CAD build for the part. Positions are in the model's coordinates, mm. Face numbers are marked on the shaded views. A direction names the side the tool comes from. Give positions to 0.01 mm unless a question says otherwise; leave off trailing zeros. Write each loop counter-clockwise with the first axis right and the second up, starting at its lowest first coordinate (ties: lowest second). Pieces come first, ordered by that corner, then holes. Notation, with made-up numbers: (6.25, 81) - (56.25, 81) arc R11 cw to (56.25, 93) - close; hole circle Ø6 at (-38, 76.25). An arc over 180 degrees is marked (long way). Put each result on its own line as item: value. Start each with the question number.
1. Mould opens along X. For the marked faces 4 and 5 say: +X half, -X half, draft (parallel to the pull), parting line (faces both ways), or undercut.
2. Tool access for the marked faces 1, 2 and 3: list every direction of +Z, -Z, +X, -X, +Y, -Y with a clear straight run to the whole face (end or side of a thin tool).
3. Cut at B-B on y = -24.45. List the corners of the cut face in (x, z).
4. Cut at C-C on x = 1.5. List the corners of the cut face in (y, z).
5. Cut at D-D on z = 9.5. List the corners of the cut face in (x, y), and give its area (3 significant figures).
6. Wall check: line 1 (X direction, y = -11.9, z = 1.75); line 2 (X direction, y = -46, z = 8.5); line 3 (X direction, y = -33.25, z = 1.55). Give the ranges that are in metal, low to high.
7. Cut at A-A on z = 16.5. List the corners of the cut face in (x, y).
8. Drop flat-ended pins along their axis: pin 1 (9.5 mm diameter, centred on x = 0, y = -52.1, fed in from -Z); pin 2 (1 mm diameter, centred on x = 17, z = 11.5, fed in from +Y); pin 3 (0.8 mm diameter, centred on y = -49.5, z = 2, fed in from +X); pin 4 (3 mm diameter, centred on x = -23.5, y = -24.45, fed in from -Z). Give the stop position or say it passes through.
Autodesk Inventor part; units mm, degrees
ref_plane "YZ Plane" through (0, 0, 0) normal (1, 0, 0) x (0, 1, 0)
ref_plane "XZ Plane" through (0, 0, 0) normal (0, 1, 0) x (-1, 0, 0)
ref_plane "XY Plane" through (0, 0, 0) normal (0, 0, 1) x (1, 0, 0)
sketch "Sketch1" plane through (0, 0, 0) normal (0, 0, 1) x (1, 0, 0)
  line L0 (-20, 0) -> (20, 0)
  line L1 (32, -12) -> (32, -47.5)
  line L2 (0, -64) -> (0, -64)
  line L3 (-32, -47.5) -> (-32, -12)
  arc A0 (-20, 0) -> (-32, -12) centre (-20, -12) ccw
  arc A1 (32, -12) -> (20, 0) centre (20, -12) ccw
  line L4 (-12, -52) -> (-12, -47.5)
  line L5 (-12, -47.5) -> (-32, -47.5)
  line L6 (12, -52) -> (12, -47.5)
  line L7 (12, -47.5) -> (32, -47.5)
  circle A2 centre (0, -52.1) radius 3.6
  line L8 (0, -80.2794) -> (0, 16.2794)
  arc A3 (-12, -52) -> (0, -64) centre (0, -52) ccw
  arc A4 (0, -64) -> (12, -52) centre (0, -52) ccw
  point P0 (0, 0)
  point P1 (0, 0)
  point P2 (0, -64)
  dimension "d0" = 64
  dimension "d1" = 64
  dimension "d2" = 12
  dimension "d3" = 47.5
  dimension "d4" = 47.5
  dimension "d5" = 7.2
  dimension "d6" = 52.1
  dimension "d8" = 12
  dimension "d9" = 12
  dimension "d10" = 12
extrude "Extrusion1" add sketch "Sketch1" along normal blind 2.5 contours L0 L8 A2 A3 L4 L5 L3 A0 | L0 A1 L1 L7 L6 A4 L8 A2
sketch "Sketch2" plane through (0, 0, 2.5) normal (0, 0, 1) x (1, 0, 0)
  line L0 (-32, -47.5) -> (-15, -47.5)
  line L1 (-15, -47.5) -> (-15, -45)
  line L2 (-15, -45) -> (-32, -45)
  line L3 (-32, -45) -> (-32, -47.5)
  line L4 (32, -47.5) -> (32, -12)
  line L5 (32, -47.5) -> (15, -47.5)
  line L6 (15, -47.5) -> (15, -45)
  line L7 (15, -45) -> (32, -45)
  line L8 (32, -45) -> (32, -47.5)
  point P0 (0, 0)
  point P1 (-12, -47.5)
  point P2 (12, -47.5)
  point P3 (32, -45)
  point P4 (15, -46.25)
  point P5 (-15, -46.25)
  dimension "d13" = 2.5
  dimension "d17" = 30
  dimension "d18" = 2.5
extrude "Extrusion2" add sketch "Sketch2" along normal blind 20.4
sketch "Sketch3" plane through (15, -45, 2.5) normal (0, 1, 0) x (1, 0, 0)
  line L0 (0, -20.4) -> (17, -20.4)
  line L1 (6.5, -20.4) -> (5, -20.4)
  line L2 (5, -20.4) -> (5, -9.4)
  line L3 (5, -9.4) -> (6.5, -9.4)
  line L4 (6.5, -9.4) -> (6.5, -20.4)
  line L5 (-3, 2.5) -> (17, 2.5)
  line L6 (-30, -20.4) -> (-47, -20.4)
  line L7 (-35, -20.4) -> (-36.5, -20.4)
  line L8 (-36.5, -20.4) -> (-36.5, -9.4)
  line L9 (-36.5, -9.4) -> (-35, -9.4)
  line L10 (-35, -9.4) -> (-35, -20.4)
  line L11 (-47, 2.5) -> (-27, 2.5)
  line L12 (0, 0) -> (0, -20.4)
  point P0 (-15, 2.5)
  point P1 (5, -14.9)
  point P2 (5, -20.4)
  dimension "d19" = 1.5
  dimension "d20" = 11.9
  dimension "d21" = 1.5
  dimension "d22" = 11.9
  dimension "d23" = 40
  dimension "d24" = 5
extrude "Extrusion3" cut sketch "Sketch3" against normal through all
fillet "Fillet1" radius 2 4 edges at (32, -46.25, 22.9) (15, -46.25, 22.9) (-15, -46.25, 22.9) (-32, -46.25, 22.9)
sketch "Sketch4" plane through (0, 0, 0) normal (0, 0, -1) x (-1, 0, 0)
  line L0 (-20, 0) -> (20, 0)
  line L1 (-32, -47.5) -> (-32, -12)
  line L2 (0, -76.8) -> (0, 12.8)
  point P0 (0, 0)
  point P1 (-20, -11.9)
  point P2 (20, -11.9)
  dimension "d28" = 11.9
  dimension "d30" = 20
  dimension "d31" = 20
hole "Hole1" at (20, -11.9, 0) at (-20, -11.9, 0) direction (0, 0, 1) diameter 5 end through all
sketch "Sketch5" plane through (0, 0, 0) normal (0, 0, -1) x (-1, 0, 0)
  line L0 (0, -76.8) -> (0, 12.8)
  line L1 (-20, 0) -> (20, 0)
  point P0 (0, 0)
  point P1 (-19, -33.25)
  point P2 (-1.5, -14.35)
  dimension "d39" = 19
  dimension "d40" = 33.25
  dimension "d41" = 1.5
  dimension "d42" = 14.35
hole "Hole2" at (19, -33.25, 0) at (1.5, -14.35, 0) direction (0, 0, 1) diameter 2.459 end through all
sketch "Sketch6" plane through (0, 0, 0) normal (0, 0, -1) x (-1, 0, 0)
  line L0 (-20, 0) -> (20, 0)
  line L1 (0, -76.8) -> (0, 12.8)
  point P0 (0, 0)
  point P1 (9.5, -24.45)
  point P2 (23.5, -24.45)
  dimension "d50" = 24.45
  dimension "d51" = 9.5
  dimension "d52" = 23.5
hole "Hole3" at (-9.5, -24.45, 0) at (-23.5, -24.45, 0) direction (0, 0, 1) diameter 2.459 end through all
sketch "Sketch7" plane through (0, 0, 0) normal (0, 0, -1) x (-1, 0, 0)
  circle A0 centre (9.5, -24.45) radius 1.2295
  circle A1 centre (9.5, -24.45) radius 2.7
  circle A2 centre (23.5, -24.45) radius 1.2295
  circle A3 centre (23.5, -24.45) radius 2.7
  point P0 (0, 0)
  dimension "d60" = 5.4
  dimension "d61" = 5.4
extrude "Extrusion4" add sketch "Sketch7" along normal blind 4.5
sketch "Sketch8" plane through (0, 0, 2.5) normal (0, 0, 1) x (1, 0, 0)
  circle A0 centre (1.5, -14.35) radius 1.2295
  circle A1 centre (1.5, -14.35) radius 2
  circle A2 centre (19, -33.25) radius 1.2295
  circle A3 centre (19, -33.25) radius 2
  point P0 (0, 0)
  dimension "d64" = 4
  dimension "d65" = 4
extrude "Extrusion5" add sketch "Sketch8" along normal blind 1.5
properties part number "Extruder Plate" material "Aluminum 6061"
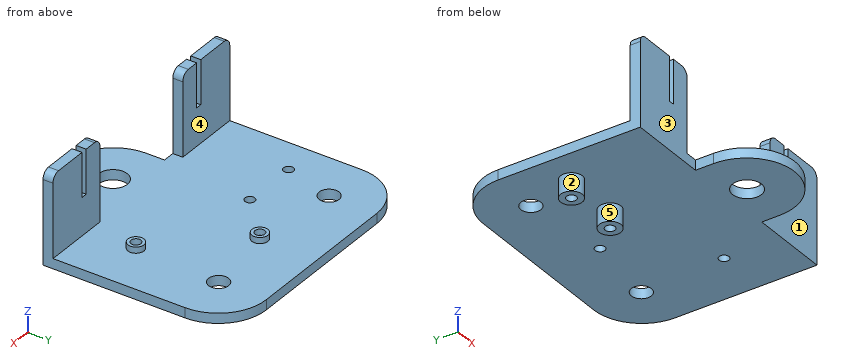
Report:
1. face 4: draft
1. face 5: undercut
2. face 1: +Z, -Z, +X, -Y
2. face 2: -Z
2. face 3: +Z, -Z, -X, -Y
3. outline: (-32, 0) - (-26.2, 0) - (-26.2, -4.5) - (-24.73, -4.5) - (-24.73, 2.5) - (-32, 2.5) - close; (-22.27, -4.5) - (-20.8, -4.5) - (-20.8, 0) - (-12.2, 0) - (-12.2, -4.5) - (-10.73, -4.5) - (-10.73, 2.5) - (-22.27, 2.5) - close; (-8.27, -4.5) - (-6.8, -4.5) - (-6.8, 0) - (32, 0) - (32, 2.5) - (-8.27, 2.5) - close
4. outline: (-63.91, 0) - (-55.37, 0) - (-55.37, 2.5) - (-63.91, 2.5) - close; (-48.83, 0) - (-15.58, 0) - (-15.58, 4) - (-16.35, 4) - (-16.35, 2.5) - (-48.83, 2.5) - close; (-13.12, 0) - (0, 0) - (0, 2.5) - (-12.35, 2.5) - (-12.35, 4) - (-13.12, 4) - close
5. outline: (-32, -47.5) - (-15, -47.5) - (-15, -45) - (-32, -45) - close; (15, -47.5) - (32, -47.5) - (32, -45) - (15, -45) - close
5. area: 85.0 mm²
6. line 1: x = -32 to -22.5, -17.5 to 17.5, 22.5 to 32
6. line 2: x = -32 to -15, 15 to 32
6. line 3: x = -32 to 17.77, 20.23 to 32
7. outline: (-32, -47.5) - (-21.5, -47.5) - (-21.5, -45) - (-32, -45) - close; (-20, -47.5) - (-15, -47.5) - (-15, -45) - (-20, -45) - close; (15, -47.5) - (20, -47.5) - (20, -45) - (15, -45) - close; (21.5, -47.5) - (32, -47.5) - (32, -45) - (21.5, -45) - close
8. pin 1: stops at z = 0
8. pin 2: stops at y = -45
8. pin 3: stops at x = 12
8. pin 4: stops at z = -4.5
